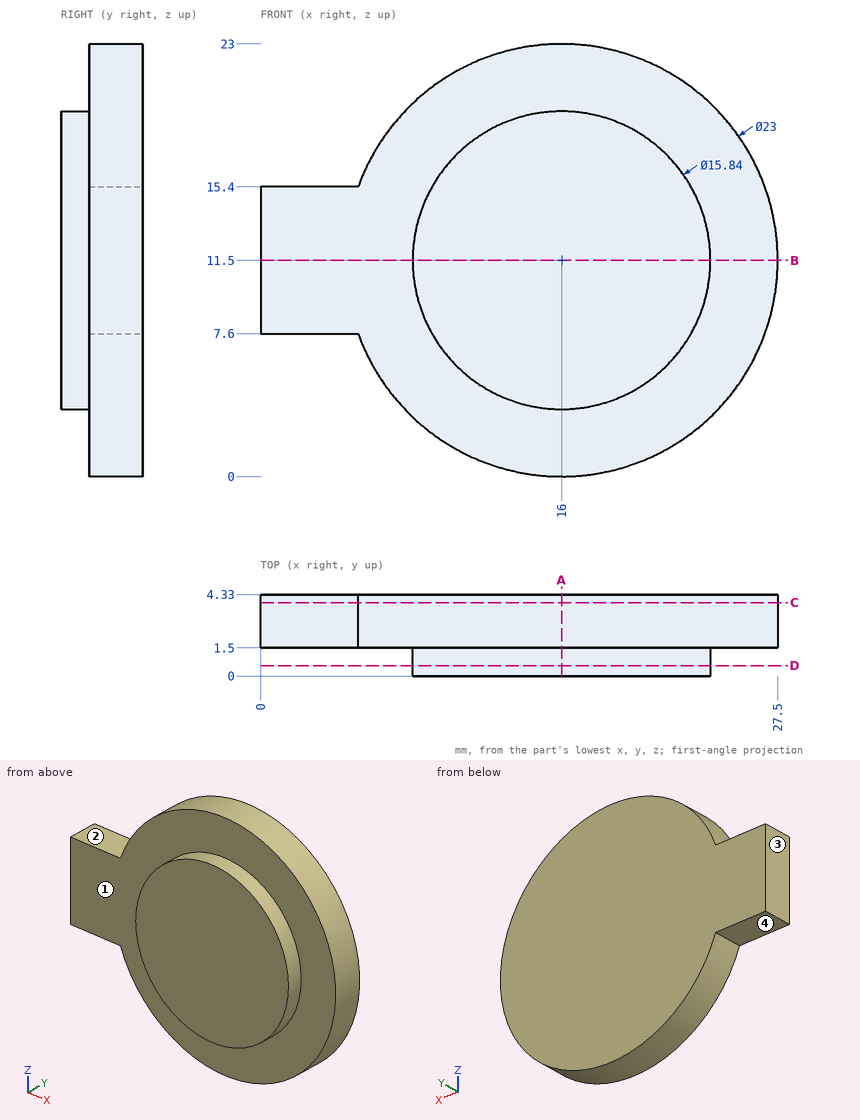
Here's the drawing with two shaded views (mm, measured from the low corner). I have some questions. A direction names the side the tool comes from. Coordinates: 2 decimals unless noted, no trailing zeros. Loops run counter-clockwise (first coordinate to the right, second up) from the corner with the lowest first, then second, coordinate; pieces in that order, holes last. Notation, with made-up numbers: (62, -0.75) -> (119, -0.75) arc R12 cw to (119, 16.25) -> close; hole circle Ø1 at (63, 24.5). An arc over 180 degrees is marked (long way). Put each result on its own line as item: value. Start each with the question number.
Q1. I want a section at B-B (z = 11.5). Write out the boundary of the cut face in (x, y), plus the area to 3 significant figures.
Q2. I want a section at C-C (y = 3.9). Write out the boundary of the cut face in (x, z), plus the area to 3 significant figures.
Q3. I want a section at A-A (x = 16). Write out the boundary of the cut face in (y, z).
Q4. For the marked faces 1, 2, 3 and 4, which set-ups out of +Z, -Z, +X, -X, +Y, -Y let a thin tool reach every point of the face, with its end or its side?
Q5. If I drill on line 1 (Y direction, x = 17.75, z = 21.5); line 2 (Z direction, x = 3, y = 3.5); line 3 (X direction, y = 2.55, z = 11.25), over which ranges is the centre line in solid material (lowest first)? Write a range as [from, to].
Q6. I want a section at D-D (y = 0.55). Write out the boundary of the cut face in (x, z).
Q7. I'm going to push flat-ended pins straight in: P1, Ø1.4, axis at x = 2, y = 2.5, coming from the +Z side; P2, Ø4, axis at x = 23.5, z = 18.5, coming from the -Y side; P3, Ø2, axis at y = 3.5, z = 15.5, coming from the +X side. Where does each tip first touch, or does it pass through?
Taken from the geometry:
1. outline: (0, 1.5) -> (8.08, 1.5) -> (8.08, 0) -> (23.92, 0) -> (23.92, 1.5) -> (27.5, 1.5) -> (27.5, 4.33) -> (0, 4.33) -> close
1. area: 102 mm2
2. outline: (0, 7.6) -> (5.18, 7.6) arc R11.5 ccw (long way) to (5.18, 15.4) -> (0, 15.4) -> close
2. area: 452 mm2
3. outline: (0, 3.58) -> (1.5, 3.58) -> (1.5, 0) -> (4.33, 0) -> (4.33, 23) -> (1.5, 23) -> (1.5, 19.42) -> (0, 19.42) -> close
4. face 1: -Y
4. face 2: +Z, -X, +Y, -Y
4. face 3: +Z, -Z, -X, +Y, -Y
4. face 4: -Z, -X, +Y, -Y
5. line 1: y = [1.5, 4.33]
5. line 2: z = [7.6, 15.4]
5. line 3: x = [0, 27.5]
6. outline: circle Ø15.84 at (16, 11.5)
7. P1: stops at z = 15.4
7. P2: stops at y = 1.5
7. P3: stops at x = 27.1
